Autodesk Inventor part; units mm, degrees
ref_plane "YZ Plane" through (0, 0, 0) normal (1, 0, 0) x (0, 1, 0)
ref_plane "XZ Plane" through (0, 0, 0) normal (0, 1, 0) x (-1, 0, 0)
ref_plane "XY Plane" through (0, 0, 0) normal (0, 0, 1) x (1, 0, 0)
sketch "Szkic1" plane through (0, 0, 0) normal (0, 1, 0) x (-1, 0, 0)
  line L0 (0, 0) -> (-15, 0)
  line L1 (-15, 0) -> (-15, -25)
  line L2 (-15, -25) -> (0, -25)
  line L3 (0, -25) -> (0, 0)
  dimension "d0" = 15
  dimension "d1" = 25
extrude "Wyciągnięcie proste1" add sketch "Szkic1" along normal blind 3
sketch "Szkic2" plane through (0, 3, 0) normal (0, 1, 0) x (1, 0, 0)
  line L0 (0, 25) -> (0, 0)
  line L1 (0, 0) -> (15, 0)
  line L2 (0, 0) -> (15, 0)
  line L3 (15, 0) -> (15, 25)
  line L4 (15, 0) -> (15, 25)
  line L5 (15, 25) -> (0, 25)
  line L6 (0, 25) -> (0, 0)
  line L7 (3.5, 4.5) -> (3.5, 20.5)
  line L8 (3.5, 20.5) -> (11.5, 20.5)
  line L9 (11.5, 20.5) -> (11.5, 4.5)
  line L10 (11.5, 4.5) -> (3.5, 4.5)
  dimension "d4" = 16
  dimension "d5" = 8
  dimension "d6" = 16
extrude "Wyciągnięcie proste2" add sketch "Szkic2" along normal blind 3
fillet "Zaokrąglenie1" radius 4 1 edges at (11.5, 4.5, -20.5)
fillet "Zaokrąglenie2" radius 4 1 edges at (3.5, 4.5, -20.5)
fillet "Zaokrąglenie3" radius 4 1 edges at (3.5, 4.5, -4.5)
fillet "Zaokrąglenie4" radius 4 1 edges at (11.5, 4.5, -4.5)
fillet "Zaokrąglenie5" radius 1 1 edges at (15, 3, -25)
fillet "Zaokrąglenie6" radius 1 1 edges at (0, 3, -25)
fillet "Zaokrąglenie7" radius 1 1 edges at (0, 3, 0)
fillet "Zaokrąglenie8" radius 1 1 edges at (15, 3, 0)
sketch "Szkic3" plane through (0, 6, 0) normal (0, 1, 0) x (1, 0, 0)
  line L0 (3, 3) -> (3, 22)
  line L1 (3, 22) -> (12, 22)
  line L2 (12, 22) -> (12, 3)
  line L3 (12, 3) -> (3, 3)
  circle A0 centre (3, 3) radius 1.5
  circle A1 centre (12, 3) radius 1.5
  circle A2 centre (12, 22) radius 1.5
  circle A3 centre (3, 22) radius 1.5
  point P0 (0, 0)
  dimension "d17" = 19
  dimension "d18" = 9
  dimension "d19" = 19
  dimension "d20" = 3
  dimension "d21" = 3
  dimension "d22" = 3
  dimension "d23" = 3
extrude "Wyciągnięcie proste3" cut sketch "Szkic3" against normal blind 6 contours L3 A0 L0 | L0 A0 L3 | A3 L1 L0 | L0 L1 A3 | A1 L2 L3 | L3 L2 A1 | A2 L2 L1 | L1 L2 A2
sketch "Szkic6" plane through (0, 0, 0) normal (0, -1, 0) x (1, 0, 0)
  circle A0 centre (11.5, -12.5) radius 2.5
  point P0 (0, 0)
  dimension "d27" = 5
extrude "Wyciągnięcie proste4" cut sketch "Szkic6" against normal blind 3
sketch "Szkic7" plane through (0, 6, 0) normal (0, 1, 0) x (1, 0, 0)
  line L0 (11.5, 16.5) -> (11.5, 8.5)
  circle A0 centre (11.5, 12.5) radius 1.5
  point P0 (0, 0)
  point P1 (11.5, 14)
  point P2 (11.5, 11)
  dimension "d30" = 3
extrude "Wyciągnięcie proste5" cut sketch "Szkic7" against normal blind 3 contours A0 L0 picked at (11.9875, 12.6113)
sketch "Szkic8" plane through (0, 0, 0) normal (0, -1, 0) x (1, 0, 0)
  circle A0 centre (7.5, -8.5) radius 2
  point P0 (0, 0)
  dimension "d33" = 4
extrude "Wyciągnięcie proste6" cut sketch "Szkic8" against normal blind 3
sketch "Szkic11" plane through (0, 0, -24) normal (-1, 0, 0) x (0, 0, 1)
  line L0 (24, 6) -> (24, 0)
  line L1 (24, 3) -> (-1, 3)
  line L2 (-1, 6) -> (-1, 0)
  line L3 (7.5, 3) -> (15.5, 3)
  line L4 (11.5, 3) -> (11.5, 6)
  line L5 (10, 6) -> (13, 6)
  line L6 (11.5, 3) -> (11.5, 0)
hole "Otwór1" at (0, 3, -12.5) direction (1, 0, 0) diameter 3 depth 3 tip angle 120
sketch "Szkic13" plane through (0, 0, -24) normal (-1, 0, 0) x (0, 0, 1)
  line L0 (9, 3) -> (14, 3)
  circle A0 centre (11.5, 3) radius 2.5
  line L1 (14, 0) -> (14, 3)
  point P0 (24, 0)
extrude "Wyciągnięcie proste7" cut sketch "Szkic13" against normal blind 1.5
Geometry check sheet. Reference: the model listing, model coordinates, mm. A direction names the side the tool comes from. Give positions to 0.01 mm unless a question says otherwise; leave off trailing zeros. Loops run counter-clockwise (first coordinate to the right, second up) from the corner with the lowest first, then second, coordinate; pieces in that order, holes last. Notation, with made-up numbers: (13.5, -9.5) -> (45.5, -9.5) arc R17 cw to (45.5, 13.5) -> close; hole circle Ø10 at (4.5, -34). An arc over 180 degrees is marked (long way). Answer in a Markdown table with one row per item. Add a question column.
1) Gauge pin test, flat ends, axial feed: P1, Ø0.8, axis at x = 13, z = -11.5, coming from the -Y side; P2, Ø6.5, axis at x = 7.5, z = -13.5, coming from the +Y side; P3, Ø2.5, axis at x = 12, z = -3, coming from the -Y side. Record the tip position at first contact, or that the pin passes through.
2) Cross-section at C-C on x = 12. Record the boundary of the cut face in (y, z), and give its area (3 significant figures).
3) Cross-section at A-A on z = -3. Record the boundary of the cut face in (x, y), and give its area (3 significant figures).
4) Cross-section at D-D on z = -12.5. Record the boundary of the cut face in (x, y).
5) Material ranges on probe 1 along X at (y, z) = (4.2, -22); probe 2 along Y at (x, z) = (2.4, -12.5); probe 3 along X at (y, z) = (4.6, -3.75), recorded low to high. Write a range as from..to.
6) Set-up check for faces 1 (the face through (4.641, 4.521, -5.703)), 2 (the face through (13.3, 3, -12.5)), 3 (the face through (1, 3, -15)): record each of +Z, -Z, +X, -X, +Y, -Y from which the full face is reachable in a straight line by a thin tool's end or side.
7) Draft check along Z on faces 4 (the face through (10.96, 1.48, -14.94)), 5 (the face through (8, 3, -12)), 6 (the face through (7, 3, 0)), 7 (the face through (14.699, 2.958, -24.715)). Enter one of: pulls with the +Z half, pulls with the -Z half, needs draft (parallel to the pull), parting line crosses it, or undercut.
8) Cross-section at B-B on x = 5.75. Record the boundary of the cut face in (y, z), and give its area (3 significant figures).
Outcome:
| question | item | result |
|---|---|---|
| 1 | P1 | stops at y = 3 |
| 1 | P2 | stops at y = 3 |
| 1 | P3 | passes through |
| 2 | outline | (0, -25) -> (6, -25) -> (6, -23.5) -> (0, -23.5) -> close; (0, -20.5) -> (6, -20.5) -> (6, -13.91) -> (3, -13.91) -> (3, -14.95) -> (0, -14.95) -> close; (0, -10.05) -> (3, -10.05) -> (3, -11.09) -> (6, -11.09) -> (6, -4.5) -> (0, -4.5) -> close; (0, -1.5) -> (6, -1.5) -> (6, 0) -> (0, 0) -> close |
| 2 | area | 90.8 mm^2 |
| 3 | outline | (0, 0) -> (1.5, 0) -> (1.5, 6) -> (0, 6) -> close; (4.5, 0) -> (10.5, 0) -> (10.5, 6) -> (4.5, 6) -> close; (13.5, 0) -> (15, 0) -> (15, 6) -> (13.5, 6) -> close |
| 3 | area | 54.0 mm^2 |
| 4 | outline | (0, 0) -> (9, 0) -> (9, 3) -> (3.87, 3) -> (3, 1.5) -> (1.5, 1.5) -> (1.5, 0.5) -> (0, 0.5) -> close; (0, 5.5) -> (1.5, 5.5) -> (1.5, 4.5) -> (3, 4.5) -> (3.5, 3.63) -> (3.5, 6) -> (0, 6) -> close; (13, 3) -> (14, 3) -> (14, 0) -> (15, 0) -> (15, 6) -> (13, 6) -> close |
| 5 | probe 1 | x = 0..1.5, 4.5..10.5, 13.5..15 |
| 5 | probe 2 | y = 0..1.5, 4.5..6 |
| 5 | probe 3 | x = 0..1.7, 4.3..10.7, 13.3..15 |
| 6 | face 1 | +Y |
| 6 | face 2 | -Y |
| 6 | face 3 | -X |
| 7 | face 4 | undercut |
| 7 | face 5 | undercut |
| 7 | face 6 | pulls with the +Z half |
| 7 | face 7 | pulls with the -Z half |
| 8 | outline | (0, -25) -> (6, -25) -> (6, -20.1) -> (3, -20.1) -> (3, -9.47) -> (0, -9.47) -> close; (0, -7.53) -> (3, -7.53) -> (3, -4.9) -> (6, -4.9) -> (6, 0) -> (0, 0) -> close |
| 8 | area | 98.6 mm^2 |
